Input: dimensioned drawing with shaded views. Units: mm. Origin: part minimum x, y, z. A direction names the side the tool comes from. Give positions to 0.01 mm unless a question says otherwise; leave off trailing zeros. Loops run counter-clockwise (first coordinate to the right, second up) from the corner with the lowest first, then second, coordinate; pieces in that order, holes last. Notation, with made-up numbers: (-38.75, 6.25) -> (-15.75, 6.25) arc R12 ccw to (-15.75, 27.25) -> close; hole circle Ø9 at (41.5, 36). An arc over 180 degrees is marked (long way). One line per question, with ' | ' between items. Start each with the question number.
Item 1: Section B-B on y = 108.5. Return loops of the section in (x, z).
Item 2: Mould query, pull axis Y, two halves, no side actions, for the marked faces 3, 4, 5 and 6. Classes: released by +Y, released by -Y, zero draft, split by the parting line, or undercut.
Item 3: Material intervals for line 1 along Y through (x, z) = (270.5, 10.5); line 2 along Y through (x, z) = (96.5, 22.5); line 3 along X through (y, z) = (36.5, 56), sorted ascending. Write a range as [from, to].
Item 4: Set-up query: the marked faces 1 and 2. Return all of +Z, -Z, +X, -X, +Y, -Y with unobstructed straight access to the full face (end or side cutting, diameter ignored); none if empty.
Item 5: Section A-A on z = 45. Return loops of the section in (x, y).
Item 6: Pin query (flat end, axial travel): P1, Ø12, axis at x = 166.5, y = 62.5, coming from the +Z side; P2, Ø6, axis at x = 16.5, y = 71.5, coming from the +Z side. Return the tip coordinate at first contact, or that it passes through.
Item 7: Section C-C on x = 141.5. Return loops of the section in (y, z), then the cut area to 3 significant figures.
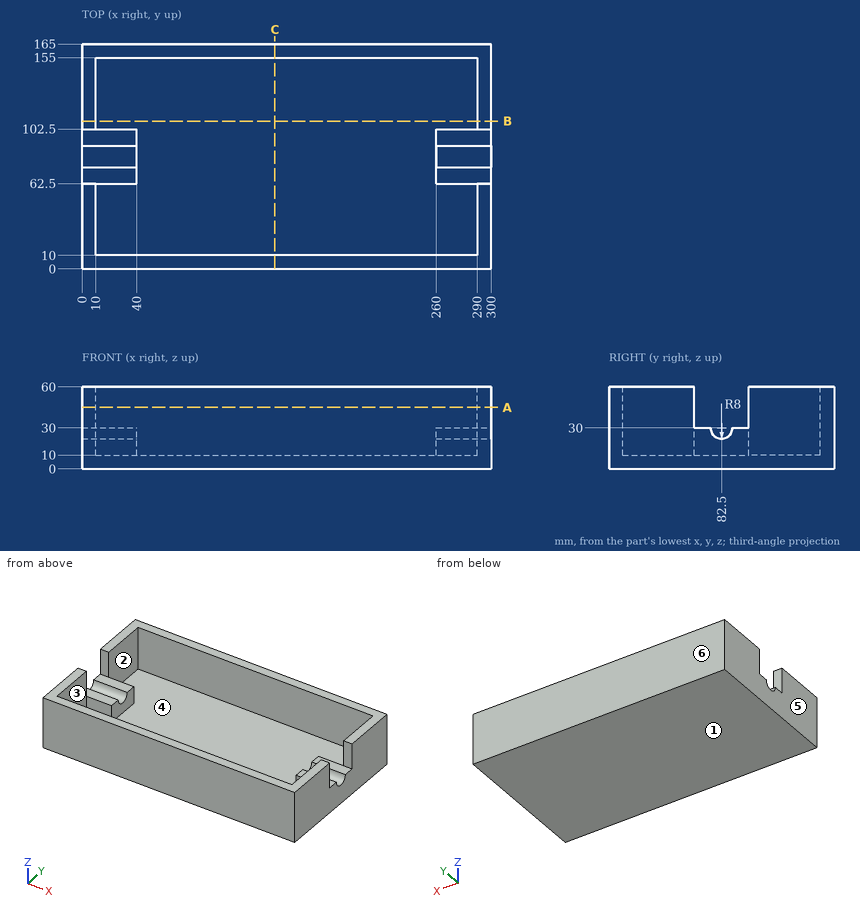
Result sheet:
1) outline: (0, 0) -> (300, 0) -> (300, 60) -> (290, 60) -> (290, 10) -> (10, 10) -> (10, 60) -> (0, 60) -> close
2) face 3: undercut | face 4: undercut | face 5: zero draft | face 6: released by +Y
3) line 1: y = [0, 10], [62.5, 102.5], [155, 165] | line 2: y = [0, 10], [155, 165] | line 3: x = [0, 10], [290, 300]
4) face 1: -Z, +X, -X, +Y, -Y | face 2: +Z
5) outline: (0, 0) -> (300, 0) -> (300, 62.5) -> (290, 62.5) -> (290, 10) -> (10, 10) -> (10, 62.5) -> (0, 62.5) -> close; (0, 102.5) -> (10, 102.5) -> (10, 155) -> (290, 155) -> (290, 102.5) -> (300, 102.5) -> (300, 165) -> (0, 165) -> close
6) P1: stops at z = 10 | P2: stops at z = 30
7) outline: (0, 0) -> (165, 0) -> (165, 60) -> (155, 60) -> (155, 10) -> (10, 10) -> (10, 60) -> (0, 60) -> close | area: 2,650 mm²
